Here's how the part is built. I have some questions about the finished solid (model axes, mm). Face numbers are marked on the shaded views. A direction names the side the tool comes from. Give positions to 0.01 mm unless a question says otherwise; leave off trailing zeros. Write each loop counter-clockwise with the first axis right and the second up, starting at its lowest first coordinate (ties: lowest second). Pieces come first, ordered by that corner, then holes. Notation, with made-up numbers: (81, 20.5) - (100, 20.5) arc R29 cw to (100, 55.5) - close; hole circle Ø11 at (-28.75, 23.25). An arc over 180 degrees is marked (long way). One line per item, written item: value. Start each with the question number.
1) On a 3-axis mill with a long thin cutter (end or side, diameter ignored), from which of +Z, -Z, +X, -X, +Y, -Y can I reach the whole of each face in a straight line? I mean the marked faces 1 and 2. Say none if no direction works.
2) Imagine slicing it at A-A on y = -3.25. Write out the boundary of the cut face in (x, z) (3 decimals), plus the area to 3 significant figures.
3) Please list where these lines run through material, in increasing order: L1, parallel to X at y = -3, z = 8 (3 decimals); L2, parallel to X at y = 1.75, z = 0 (3 decimals); L3, parallel to Y at x = 12, z = 6. Write a range as [from, to].
4) I'm going to push flat-ended pins straight in: P1, Ø8, axis at x = -52, z = 17.5, coming from the -Y side; P2, Ø2.5, axis at y = -3.5, z = 2.5, coming from the -X side (3 decimals); P3, Ø3, axis at y = -2, z = 4, coming from the +X side (3 decimals); P4, Ø4.5, axis at x = 0, z = 0, coming from the +Y side. Where does each tip first touch, or does it pass through?
5) Imagine slicing it at B-B on x = 0. Write out the boundary of the cut face in (y, z) (3 decimals), plus the area to 3 significant figures.
6) We'd pull the mould along X, two halves only. Please class the marked faces 3, 4 and 5: +X half, -X half, draft (parallel to the pull), parting line (faces both ways), or undercut.
7) Imagine slicing it at C-C on z = 18. Write out the boundary of the cut face in (x, y).
8) Imagine slicing it at D-D on y = 2. Write out the boundary of the cut face in (x, z) (3 decimals), plus the area to 3 significant figures.
from build123d import *

# Parameters (mm, degrees)
SKETCH1_R           = 8.89
SKETCH1_R_2         = 3.925
BOSS_EXTRUDE1_DEPTH = 6.35
SKETCH2_W           = 12.7
SKETCH2_H           = 0.6
CUT_EXTRUDE1_DEPTH  = 143.733819135
SKETCH3_W           = 3.0988
SKETCH3_H           = 19.05
BOSS_EXTRUDE2_DEPTH = 6.35
FILLET4_R           = 10
FILLET1_R           = 3
FILLET2_R           = 1


with BuildPart() as part:
    # Sketch1 → Boss-Extrude1 (new body)
    # profile 1 of 2: a face of its own
    with BuildSketch(Plane(origin=(0, 0, 0), x_dir=(1, 0, 0), z_dir=(0, 1, 0))):
        Polygon((-69.85, -28.575), (69.85, -28.575), (69.85, -9.525), (22.225, -9.525), (22.225, 9.525), (-22.225, 9.525), (-22.225, -9.525), (-69.85, -9.525), align=None)
        Circle(SKETCH1_R, mode=Mode.SUBTRACT)
    # profile 2 of 2: a face of its own
    with BuildSketch(Plane(origin=(0, 0, 0), x_dir=(1, 0, 0), z_dir=(0, 1, 0))):
        Circle(SKETCH1_R)
        with Locations(Location((0, 0, 0), (0, 0, 270))):
            Circle(SKETCH1_R_2, mode=Mode.SUBTRACT)
    extrude(amount=BOSS_EXTRUDE1_DEPTH)

    # Sketch2 → Cut-Extrude1 (cut, through all)
    with BuildSketch(Plane(origin=(69.85, 0, 0), x_dir=(0, 0, -1), z_dir=(1, 0, 0))):
        with Locations((-22.225, 0.3)):
            Rectangle(SKETCH2_W, SKETCH2_H)
    extrude(amount=-CUT_EXTRUDE1_DEPTH, mode=Mode.SUBTRACT)

    # Sketch3 → Boss-Extrude2 (add)
    with BuildSketch(Plane.XZ):
        with Locations((-20.6756, 0)):
            Rectangle(SKETCH3_W, SKETCH3_H)
    boss_extrude2 = extrude(amount=BOSS_EXTRUDE2_DEPTH)

    # Mirror1: Boss-Extrude2 across plane
    add(boss_extrude2.mirror(Plane(origin=(0, 0, 0), x_dir=(0, 0, 1), z_dir=(1, 0, 0))))

    # Fillet4
    fillet4_edges = [part.edges().sort_by_distance(p)[0] for p in [
        (-22.225, 3.175, 9.525),
        (22.225, 3.175, 9.525),
    ]]
    fillet(fillet4_edges, radius=FILLET4_R)

    # Fillet1
    fillet1_edges = [part.edges().sort_by_distance(p)[0] for p in [
        (0, 6.35, 28.575),
        (69.85, 6.35, 19.05),
        (0, 6.35, -9.525),
        (-51.0375, 6.35, 9.525),
        (-69.85, 6.35, 19.05),
        (22.225, 6.35, -5),
        (51.0375, 6.35, 9.525),
        (-22.225, 6.35, -5),
        (25.153932188, 6.35, 6.596067812),
        (-25.153932188, 6.35, 6.596067812),
    ]]
    fillet(fillet1_edges, radius=FILLET1_R)

    # Fillet2
    fillet2_edges = [part.edges().sort_by_distance(p)[0] for p in [
        (-19.1262, 0, 0),
        (19.1262, 0, 0),
    ]]
    fillet(fillet2_edges, radius=FILLET2_R)


solid = part.part
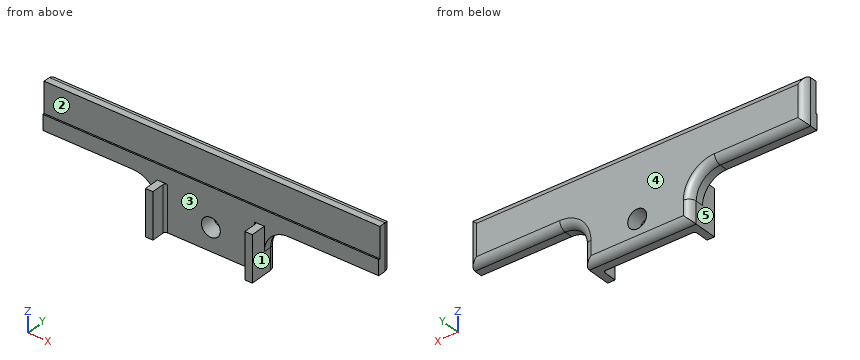
Numbers:
1. face 1: -Z, +X, -Y
1. face 2: +Z, +X, -X, -Y
2. outline: (-22.225, -9.525) - (-19.126, -9.525) - (-19.126, 9.525) - (-22.225, 9.525) - close; (19.126, -9.525) - (22.225, -9.525) - (22.225, 9.525) - (19.126, 9.525) - close
2. area: 118 mm^2
3. L1: [-22.225, -19.126], [19.126, 22.225]
3. L2: [-22.236, -3.925], [3.925, 22.236]
3. L3: [0, 6.35]
4. P1: y = 0
4. P2: x = -22.225
4. P3: x = 22.225
4. P4: through
5. outline: (0, -9.525) - (3.35, -9.525) arc R3 ccw to (6.35, -6.525) - (6.35, -3.925) - (0, -3.925) - close; (0, 3.925) - (6.35, 3.925) - (6.35, 25.575) arc R3 ccw to (3.35, 28.575) - (0.6, 28.575) - (0.6, 15.875) - (0, 15.875) - close
5. area: 181 mm^2
6. face 3: undercut
6. face 4: draft
6. face 5: -X half
7. outline: (-69.85, 0.6) - (69.85, 0.6) - (69.85, 3.35) arc R3 ccw to (66.85, 6.35) - (-66.85, 6.35) arc R3 ccw to (-69.85, 3.35) - close
8. outline: (-69.85, 9.525) - (-32.225, 9.525) arc R10 cw to (-22.225, -0.475) - (-22.225, -9.525) - (22.225, -9.525) - (22.225, -0.475) arc R10 cw to (32.225, 9.525) - (69.85, 9.525) - (69.85, 28.575) - (-69.85, 28.575) - close; hole circle Ø7.85 at (0, 0)
8. area: 3,500 mm^2
